Read the model definition and answer for the solid it produces. Units are mm, in the model's axes. A direction names the side the tool comes from. Round coordinates to 2 decimals unless told otherwise and drop trailing zeros. Write each loop counter-clockwise with the first axis right and the second up, starting at its lowest first coordinate (ties: lowest second). Pieces come first, ordered by that corner, then holes. Notation, with made-up numbers: (65, 71) - (89, 71) arc R24 ccw to (89, 100) - close; hole circle Ø8 at (-25.5, -38). An arc over 180 degrees is marked (long way). Answer as CSV lines item,"result". Start each with the question number.
1) Find section C-C on y = 18. Determine the outline of the cut face in (x, z).
2) For a pull along Z with two mould halves and no side action, classify faces 5 (the flat face through (0, 15.273, 5)), 6 (the cylindrical face through (0.02, 9.06, 5.23)), 7 (the flat face through (0, 16, -2)) as +Z half, -Z half, draft (parallel to the pull), parting line (faces both ways), or undercut.
3) Find section D-D on y = 0. Determine the outline of the cut face in (x, z), then the cut area to 3 significant figures.
4) Each of these flat-tipped pins is pushed along its axis until it touches: pin 1 (2 mm diameter, centred on x = -0.5, z = 5.5, fed in from +Y); pin 2 (7 mm diameter, centred on y = -5.5, z = 1.5, fed in from -X); pin 3 (4 mm diameter, centred on y = 0, z = -4, fed in from +X). Where does it stop, or does it pass through?
5) Find section A-A on x = 0. Determine the outline of the cut face in (y, z).
6) Which of the six approach directions +Z, -Z, +X, -X, +Y, -Y give full straight-line access (tool end or side, diameter ignored) to faces 1 (the flat face through (1.25, 1, 0)), 2 (the flat face through (0, 16, 2)), 3 (the flat face through (-1.25, 1, 0)), 4 (the flat face through (0, 15.273, -4))?
7) Find section B-B on z = -4. Determine the outline of the cut face in (x, y), then the cut area to 3 significant figures.
8) Consider line 1 along Y through (x, z) = (0.05, -4); line 2 along Z through (x, y) = (0.2, -10); line 3 along X through (y, z) = (12.5, 1). Determine where each line is inside the solid, lowest interval first.
from build123d import *

# Parameters (mm, degrees)
SKETCH2_W           = 2.5
SKETCH2_H           = 28.272821971
BOSS_EXTRUDE5_DEPTH = 7
SKETCH2_8_R         = 3
BOSS_EXTRUDE6_DEPTH = 2
SKETCH3_R           = 1.7
CUT_EXTRUDE1_DEPTH  = 24.043437244
SKETCH4_R           = 1.55
CUT_EXTRUDE2_DEPTH  = 23.540241791


with BuildPart() as part:
    # Sketch2 → Boss-Extrude5 (new, symmetric)
    with BuildSketch(Plane.XY):
        with Locations((0, 1.136410986)):
            Rectangle(SKETCH2_W, SKETCH2_H)
    extrude(amount=BOSS_EXTRUDE5_DEPTH, both=True)

    # Sketch2_8 → Boss-Extrude6 (add, symmetric)
    with BuildSketch(Plane.XY):
        with Locations((0, 18)):
            Circle(SKETCH2_8_R)
    extrude(amount=BOSS_EXTRUDE6_DEPTH, both=True)

    # Sketch3 → Cut-Extrude1 (cut, through all)
    with BuildSketch(Plane.XY.offset(2)):
        with Locations((0, 18)):
            Circle(SKETCH3_R)
    extrude(amount=-CUT_EXTRUDE1_DEPTH, mode=Mode.SUBTRACT)

    # Sketch4 → Cut-Extrude2 (cut, through all)
    with BuildSketch(Plane(origin=(1.25, 0, 0), x_dir=(0, 0, -1), z_dir=(1, 0, 0))):
        with Locations((4, 0)):
            Circle(SKETCH4_R)
        with Locations((-4, 0)):
            Circle(SKETCH4_R)
        with Locations((-4, 10)):
            Circle(SKETCH4_R)
        with Locations((4, 10)):
            Circle(SKETCH4_R)
        with Locations(Location((4, -10, 0), (0, 0, 180))):
            Circle(SKETCH4_R)
        with Locations(Location((-4, -10, 0), (0, 0, 180))):
            Circle(SKETCH4_R)
    extrude(amount=-CUT_EXTRUDE2_DEPTH, mode=Mode.SUBTRACT)


solid = part.part
Check values:
1,outline,"(-3, -2) - (-1.7, -2) - (-1.7, 2) - (-3, 2) - close; (1.7, -2) - (3, -2) - (3, 2) - (1.7, 2) - close"
2,face 5,"draft"
2,face 6,"undercut"
2,face 7,"-Z half"
3,outline,"(-1.25, -7) - (1.25, -7) - (1.25, -5.55) - (-1.25, -5.55) - close; (-1.25, -2.45) - (1.25, -2.45) - (1.25, 2.45) - (-1.25, 2.45) - close; (-1.25, 5.55) - (1.25, 5.55) - (1.25, 7) - (-1.25, 7) - close"
3,area,"19.5 mm^2"
4,pin 1,"stops at y = 15.27"
4,pin 2,"stops at x = -1.25"
4,pin 3,"stops at x = 1.25"
5,outline,"(-13, -7) - (15.27, -7) - (15.27, -2) - (16.3, -2) - (16.3, 2) - (15.27, 2) - (15.27, 7) - (-13, 7) - close; (19.7, -2) - (21, -2) - (21, 2) - (19.7, 2) - close; hole circle Ø3.1 at (-10, -4); hole circle Ø3.1 at (-10, 4); hole circle Ø3.1 at (0, -4); hole circle Ø3.1 at (0, 4); hole circle Ø3.1 at (10, -4); hole circle Ø3.1 at (10, 4)"
6,face 1,"+Z, -Z, +X, -Y"
6,face 2,"+Z, +X, -X, +Y"
6,face 3,"+Z, -Z, -X, -Y"
6,face 4,"-Z, +X, -X, +Y"
7,outline,"(-1.25, -13) - (1.25, -13) - (1.25, -11.55) - (-1.25, -11.55) - close; (-1.25, -8.45) - (1.25, -8.45) - (1.25, -1.55) - (-1.25, -1.55) - close; (-1.25, 1.55) - (1.25, 1.55) - (1.25, 8.45) - (-1.25, 8.45) - close; (-1.25, 11.55) - (1.25, 11.55) - (1.25, 15.27) - (-1.25, 15.27) - close"
7,area,"47.4 mm^2"
8,line 1,"y = -13 to -11.55, -8.45 to -1.55, 1.55 to 8.45, 11.55 to 15.27"
8,line 2,"z = -7 to -5.55, -2.45 to 2.45, 5.55 to 7"
8,line 3,"x = -1.25 to 1.25"
